Read the model definition and answer for the solid it produces. Units are mm, in the model's axes. Coordinates: 2 decimals unless noted, no trailing zeros. Loops run counter-clockwise (first coordinate to the right, second up) from the corner with the lowest first, then second, coordinate; pieces in that order, holes last. Notation, with made-up numbers: (89, -5.5) - (95, -5.5) arc R25 cw to (95, 12.5) - close; hole circle Ø5 at (62.5, 41). An arc over 180 degrees is marked (long way). One line per item, written item: value. Start each with the question number.
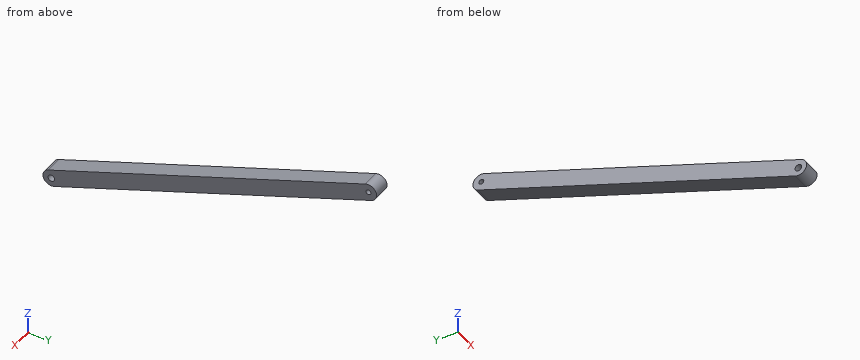
from build123d import *

# Parameters (mm, degrees)
BOSS_EXTRUDE1_DEPTH      = 5
BOSS_EXTRUDE1_DEPTH_BACK = 5
SKETCH2_R                = 1.5
SKETCH2_R_2              = 2


with BuildPart() as part:
    # Sketch2 → Boss-Extrude1 (new, two sides: drawn at the far end of the back side and taken through both)
    with BuildSketch(Plane(origin=(0, 0, 0), x_dir=(0, 0, -1), z_dir=(1, 0, 0)).offset(-BOSS_EXTRUDE1_DEPTH_BACK)):
        with BuildLine():
            Line((-37.711923347, -132.743444835), (-111.443355455, 58.568457266))
            ThreePointArc((-111.443355455, 58.568457266), (-108.575933735, 65.032039298), (-102.112351703, 62.164617578))
            Line((-102.112351703, 62.164617578), (-28.380919596, -129.147284523))
            ThreePointArc((-28.380919596, -129.147284523), (-31.248341316, -135.610866555), (-37.711923347, -132.743444835))
        make_face()
        with Locations((-106.777853579, 60.366537422)):
            Circle(SKETCH2_R, mode=Mode.SUBTRACT)
        with Locations((-33.046421472, -130.945364679)):
            Circle(SKETCH2_R_2, mode=Mode.SUBTRACT)
    extrude(amount=BOSS_EXTRUDE1_DEPTH + BOSS_EXTRUDE1_DEPTH_BACK)


solid = part.part
1) Flat-ended cylindrical pins translate along their axes: P1, Ø1, axis at x = -1, y = -72.5, coming from the +Z side; P2, Ø4, axis at x = -3.5, y = 27, coming from the +Z side. Find the tip coordinate at first contact, or state that the pin passes through.
2) Section C-C, the plane z = 74 is taken. Determine the outline of the cut face in (x, y), and give its area (3 significant figures).
3) Straight lines are drawn through the part: L1, parallel to Z at x = 1.5, y = -108; L2, parallel to Z at x = -4.5, y = -33.5. For each, find the intervals that lie inside material, in ascending order.
4) Section A-A, the plane x = -0.25 is taken. Determine the outline of the cut face in (y, z).
5) Section B-B, the plane y = -19.5 is taken. Determine the outline of the cut face in (x, z), and give its area (3 significant figures).
Answer below:
1. P1: z = 61.12
1. P2: z = 100.05
2. outline: (-5, -38.59) - (5, -38.59) - (5, -10.78) - (-5, -10.78) - close
2. area: 278 mm2
3. L1: 36.53 to 47.25
3. L2: 65.24 to 75.96
4. outline: (-132.74, 37.71) arc R5 ccw to (-129.15, 28.38) - (62.16, 102.11) arc R5 ccw to (58.57, 111.44) - close; hole circle Ø4 at (-130.95, 33.05); hole circle Ø3 at (60.37, 106.78)
5. outline: (-5, 70.64) - (5, 70.64) - (5, 81.36) - (-5, 81.36) - close
5. area: 107 mm2
